```python
from build123d import *

# Parameters (mm, degrees)
BOSS_EXTRUDE1_DEPTH = 12.5
SKETCH2_R           = 2
CUT_EXTRUDE1_DEPTH  = 8


with BuildPart() as part:
    # Sketch1 → Boss-Extrude1 (new body)
    with BuildSketch(Plane.XY):
        Polygon((0, 0), (0, -17), (50, -17), (50, -13), (30, 0), align=None)
    extrude(amount=BOSS_EXTRUDE1_DEPTH)

    # Sketch2 → Cut-Extrude1 (cut)
    with BuildSketch(Plane(origin=(0, 0, 0), x_dir=(1, 0, 0), z_dir=(0, 1, 0))):
        with Locations((6.5, -6.25)):
            Circle(SKETCH2_R)
        with Locations((23.5, -6.25)):
            Circle(SKETCH2_R)
    extrude(amount=-CUT_EXTRUDE1_DEPTH, mode=Mode.SUBTRACT)


solid = part.part
```
Design review of the part built by this model. Coordinates are the model's own, in mm. A direction names the side the tool comes from. Coordinates: 2 decimals unless noted, no trailing zeros. Order: outer loops, then holes, each group sorted by start corner. A loop starts at its lowest first (then second) coordinate and runs counter-clockwise, first axis right, second up. Notation, with made-up numbers: M 44.5,-16.75 L 66.5,-16.75 A14 cw 66.5,1.25 Z; hole C 22,81.5 d4. An arc over 180 degrees is marked long. Answer as a JSON object with one key per item and string values. Group by question number.
1) For pin 1 (6 mm diameter, centred on y = -3, z = 6.5, fed in from +X), flat-tipped, find the tip position at first contact; note if it passes through.
2) Add section C-C, the plane y = -4. Write out the cut boundary in (x, z), then the cut area to 3 significant figures.
3) Wall thickness on L1, parallel to X at y = -4.25, z = 6.25; L2, parallel to X at y = -2.5, z = 6.25; L3, parallel to Z at x = 23.5, y = -2: over which ranges is each line inside the solid? List them lowest first.
4) Add section B-B, the plane z = 8.75. Write out the cut boundary in (x, y).
5) Add section A-A, the plane x = 6.5. Write out the cut boundary in (y, z), then the cut area to 4 significant figures.
6) Tool access review of faces 4 (the cylindrical face through (4.913, -3.944, 7.467)), 5 (the flat face through (25, -17, 6)): name each direction out of +Z, -Z, +X, -X, +Y, -Y from which nothing blocks a thin tool from reaching the whole face with its end or side.
7) Mouldability with a two-part tool opening along X and no side actions: class faces 1 (the flat face through (0, -8, 6)), 2 (the flat face through (50, -15, 6)), 3 (the cylindrical face through (21.5, -3.9, 6.2)) as pulls with the +X half, pulls with the -X half, needs draft (parallel to the pull), parting line crosses it, or undercut.
8) Add section D-D, the plane z = 6.25. Write out the cut boundary in (x, y), then the cut area to 3 significant figures.
Computed values:
{
 "1": {"pin 1": "stops at x = 39.23"},
 "2": {"outline": "M 0,0 L 36.15,0 L 36.15,12.5 L 0,12.5 Z; hole C 6.5,6.25 d4; hole C 23.5,6.25 d4", "area": "427 mm^2"},
 "3": {"L1": "x = 0 to 4.5, 8.5 to 21.5, 25.5 to 36.54", "L2": "x = 0 to 4.5, 8.5 to 21.5, 25.5 to 33.85", "L3": "z = 0 to 4.25, 8.25 to 12.5"},
 "4": {"outline": "M 0,-17 L 50,-17 L 50,-13 L 30,0 L 0,0 Z"},
 "5": {"outline": "M -17,0 L 0,0 L 0,4.25 L -8,4.25 L -8,8.25 L 0,8.25 L 0,12.5 L -17,12.5 Z", "area": "180.5 mm^2"},
 "6": {"face 4": "+Y", "face 5": "+Z, -Z, +X, -X, -Y"},
 "7": {"face 1": "pulls with the -X half", "face 2": "pulls with the +X half", "face 3": "undercut"},
 "8": {"outline": "M 0,-17 L 50,-17 L 50,-13 L 30,0 L 25.5,0 L 25.5,-8 L 21.5,-8 L 21.5,0 L 8.5,0 L 8.5,-8 L 4.5,-8 L 4.5,0 L 0,0 Z", "area": "656 mm^2"}
}
